Read the model definition and answer for the solid it produces. Units are mm, in the model's axes. Coordinates: 2 decimals unless noted, no trailing zeros. Order: outer loops, then holes, each group sorted by start corner. A loop starts at its lowest first (then second) coordinate and runs counter-clockwise, first axis right, second up. Notation, with made-up numbers: M 22,-38 L 72,-38 A31 cw 72,-8 Z; hole C 89.25,70 d10. An arc over 180 degrees is marked long. Put each result on its own line as item: value.
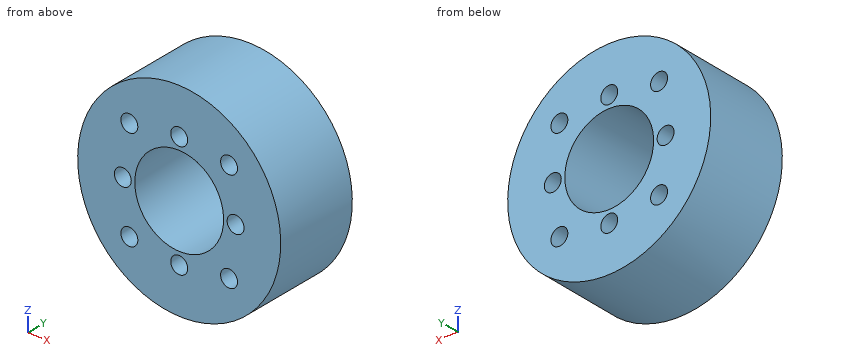
from build123d import *

# Parameters (mm, degrees)
SKETCH1_R           = 36
BOSS_EXTRUDE1_DEPTH = 30
SKETCH2_R           = 3
CUT_EXTRUDE1_DEPTH  = 30
SKETCH4_R           = 3
CUT_EXTRUDE2_DEPTH  = 30
SKETCH5_R           = 15.75
CUT_EXTRUDE3_DEPTH  = 30


with BuildPart() as part:
    # Sketch1 → Boss-Extrude1 (new body)
    with BuildSketch(Plane(origin=(0, 0, 0), x_dir=(1, 0, 0), z_dir=(0, 1, 0))):
        with Locations(Location((0, 0, 0), (0, 0, 270))):
            Circle(SKETCH1_R)
    extrude(amount=BOSS_EXTRUDE1_DEPTH)

    # Sketch2 → Cut-Extrude1 (cut)
    with BuildSketch(Plane(origin=(0, 30, 0), x_dir=(1, 0, 0), z_dir=(0, 1, 0))):
        with Locations(Location((20, 0, 0), (0, 0, 270))):
            Circle(SKETCH2_R)
        with Locations(Location((0, -20, 0), (0, 0, 270))):
            Circle(SKETCH2_R)
        with Locations(Location((-20, 0, 0), (0, 0, 270))):
            Circle(SKETCH2_R)
        with Locations(Location((0, 20, 0), (0, 0, 270))):
            Circle(SKETCH2_R)
    extrude(amount=-CUT_EXTRUDE1_DEPTH, mode=Mode.SUBTRACT)

    # Sketch4 → Cut-Extrude2 (cut)
    with BuildSketch(Plane(origin=(0, 30, 0), x_dir=(1, 0, 0), z_dir=(0, 1, 0))):
        with Locations(Location((17.67766953, 17.67766953, 0), (0, 0, 270))):
            Circle(SKETCH4_R)
        with Locations(Location((17.67766953, -17.67766953, 0), (0, 0, 270))):
            Circle(SKETCH4_R)
        with Locations(Location((-17.67766953, -17.67766953, 0), (0, 0, 270))):
            Circle(SKETCH4_R)
        with Locations(Location((-17.67766953, 17.67766953, 0), (0, 0, 270))):
            Circle(SKETCH4_R)
    extrude(amount=-CUT_EXTRUDE2_DEPTH, mode=Mode.SUBTRACT)

    # Sketch5 → Cut-Extrude3 (cut)
    with BuildSketch(Plane(origin=(0, 30, 0), x_dir=(1, 0, 0), z_dir=(0, 1, 0))):
        with Locations(Location((0, 0, 0), (0, 0, 270))):
            Circle(SKETCH5_R)
    extrude(amount=-CUT_EXTRUDE3_DEPTH, mode=Mode.SUBTRACT)


solid = part.part
Q1. Consider line 1 along X through (y, z) = (22.5, 16.5); line 2 along X through (y, z) = (7.25, 20); line 3 along Z through (x, y) = (2.5, 26). Determine where each line is inside the solid, lowest interval first.
Answers below:
line 1: x = -32 to -20.44, -14.92 to 14.92, 20.44 to 32
line 2: x = -29.93 to -19.58, -15.78 to -3, 3 to 15.78, 19.58 to 29.93
line 3: z = -35.91 to -21.66, -18.34 to -15.55, 15.55 to 18.34, 21.66 to 35.91
Q2. Given pin 1 (19 mm diameter, centred on x = 0, z = 0, fed in from -Y); pin 2 (10 mm diameter, centred on x = -21.5, y = 18.5, fed in from +Z); pin 3 (2 mm diameter, centred on y = 17, z = 16.5, fed in from +X); pin 4 (10 mm diameter, centred on y = 8, z = 21.5, fed in from -X), each flat-ended and moving along its own axis, determine where each tip first touches the part or whether it passes through.
Answers below:
pin 1: passes through
pin 2: stops at z = 32
pin 3: stops at x = 32.49
pin 4: stops at x = -32
Q3. Find section B-B on z = 0. Write down the section's boundary in (x, y), plus the area to 3 significant figures.
Answers below:
outline: M -36,0 L -23,0 L -23,30 L -36,30 Z; M -17,0 L -15.75,0 L -15.75,30 L -17,30 Z; M 15.75,0 L 17,0 L 17,30 L 15.75,30 Z; M 23,0 L 36,0 L 36,30 L 23,30 Z
area: 855 mm^2
Q4. Find section D-D on y = 2. Give the number of separate pieces and of enclosed holes in the cut face, plus the area to 3 significant figures.
Answers below:
separate pieces: 1
enclosed holes: 9
area: 3,070 mm^2
Q5. Find section A-A on x = 0. Write down the section's boundary in (y, z).
Answers below:
outline: M 0,-36 L 30,-36 L 30,-23 L 0,-23 Z; M 0,-17 L 30,-17 L 30,-15.75 L 0,-15.75 Z; M 0,15.75 L 30,15.75 L 30,17 L 0,17 Z; M 0,23 L 30,23 L 30,36 L 0,36 Z
Q6. Find section C-C on z = -11.5. Write down the section's boundary in (x, y).
Answers below:
outline: M -34.11,0 L -10.76,0 L -10.76,30 L -34.11,30 Z; M 10.76,0 L 34.11,0 L 34.11,30 L 10.76,30 Z
